Here's how the part is built. I have some questions about the finished solid (model axes, mm). Face numbers are marked on the shaded views. A direction names the side the tool comes from. Give positions to 0.01 mm unless a question says otherwise; leave off trailing zeros. Write each loop counter-clockwise with the first axis right and the second up, starting at its lowest first coordinate (ties: lowest second). Pieces come first, ordered by that corner, then holes. Notation, with made-up numbers: (79.25, 54.25) - (86.25, 54.25) arc R20 cw to (86.25, 73.25) - close; hole circle Ø6 at (42, 22.5). An arc over 180 degrees is marked (long way). Write each question's results on one line, items separated by ' | '. Start each with the question number.
Item 1: We'd pull the mould along Y, two halves only. Please class the marked faces 1, 2, 3 and 4: +Y half, -Y half, draft (parallel to the pull), parting line (faces both ways), or undercut.
Item 2: Suppose I cut it at A-A on z = 3.5. List the corners of the cut face in (x, y) for me, then the cut area to 3 significant figures.
Item 3: Which directions (+Z, -Z, +X, -X, +Y, -Y) give clear straight access to the entire face, cutting with the end or side of a thin tool? Please do the marked faces 5 and 6.
Item 4: Will these pins go through, and if not, where does the flat tip stop? P1, Ø15, axis at x = 18, y = 31, coming from the -Z side; P2, Ø8, axis at x = 23.5, y = 22.5, coming from the -Z side; P3, Ø2.5, axis at x = 15.5, y = 8, coming from the -Z side.
Item 5: Suppose I cut it at C-C on y = 13.5. List the corners of the cut face in (x, z) for me, then the cut area to 3 significant figures.
Item 6: Suppose I cut it at B-B on x = 26. List the corners of the cut face in (y, z) for me, then the cut area to 3 significant figures.
Item 7: Please list where these lines run through material, in increasing order: line 1 along Y through (x, z) = (11.5, 12); line 2 along X through (y, z) = (18, 6.5); line 3 along Y through (x, z) = (27, 8.5).
```python
from build123d import *

# Parameters (mm, degrees)
SKETCH_1_W          = 33
SKETCH_1_H          = 44
EXTRUDE_1_DEPTH     = 12.5
SKETCH_2_W          = 29.6
SKETCH_2_H          = 40.6
CUT_EXTRUDE_2_DEPTH = 11
SKETCH_3_W          = 27.6
SKETCH_3_H          = 31.1
CUT_EXTRUDE_3_DEPTH = 2.5
SKETCH_4_W          = 18
SKETCH_4_H          = 3
CUT_EXTRUDE_4_DEPTH = 0.7
FILLET_1_R          = 1
SKETCH_5_W          = 27.6
SKETCH_5_H          = 0.6
EXTRUDE_2_DEPTH     = 1
EXTRUDE_3_DEPTH     = 8
EXTRUDE_4_DEPTH     = 0.6
SKETCH_8_W          = 27.6
SKETCH_8_H          = 27.1
CUT_EXTRUDE_5_DEPTH = 1.6
CUT_EXTRUDE_6_DEPTH = 5


with BuildPart() as part:
    # 草图1 → 凸台-拉伸1 (new body)
    with BuildSketch(Plane.XY):
        with Locations((16.5, 22)):
            Rectangle(SKETCH_1_W, SKETCH_1_H)
    extrude(amount=EXTRUDE_1_DEPTH)

    # 草图2 → 切除-拉伸2 (cut)
    with BuildSketch(Plane(origin=(0, 0, 0), x_dir=(-1, 0, 0), z_dir=(0, 0, -1))):
        with Locations((-16.5, 22)):
            Rectangle(SKETCH_2_W, SKETCH_2_H)
    extrude(amount=-CUT_EXTRUDE_2_DEPTH, mode=Mode.SUBTRACT)

    # 草图3 → 切除-拉伸3 (cut, through all)
    with BuildSketch(Plane(origin=(0, 0, 11), x_dir=(-1, 0, 0), z_dir=(0, 0, -1))):
        with Locations((-16.5, 21.75)):
            Rectangle(SKETCH_3_W, SKETCH_3_H)
    extrude(amount=-CUT_EXTRUDE_3_DEPTH, mode=Mode.SUBTRACT)

    # 草图4 → 切除-拉伸4 (cut)
    with BuildSketch(Plane(origin=(0, 0, 11), x_dir=(-1, 0, 0), z_dir=(0, 0, -1))):
        with Locations((-16.5, 40.8)):
            Rectangle(SKETCH_4_W, SKETCH_4_H)
    extrude(amount=-CUT_EXTRUDE_4_DEPTH, mode=Mode.SUBTRACT)

    # 圆角1
    fillet_1_edges = [part.edges().sort_by_distance(p)[0] for p in [
        (0, 44, 6.25),
        (33, 44, 6.25),
        (33, 0, 6.25),
        (0, 0, 6.25),
    ]]
    fillet(fillet_1_edges, radius=FILLET_1_R)

    # 草图5 → 凸台-拉伸2 (add)
    with BuildSketch(Plane(origin=(0, 6.2, 0), x_dir=(1, 0, 0), z_dir=(0, 1, 0))):
        with Locations((16.5, -12.2)):
            Rectangle(SKETCH_5_W, SKETCH_5_H)
    extrude(amount=EXTRUDE_2_DEPTH)

    # 草图6 → 凸台-拉伸3 (add)
    with BuildSketch(Plane(origin=(0, 0, 11), x_dir=(-1, 0, 0), z_dir=(0, 0, -1))):
        with BuildLine():
            Line((-31.3, 11.6), (-31.3, 12.4))
            ThreePointArc((-31.3, 12.4), (-30.9, 12), (-31.3, 11.6))
        make_face()
        with BuildLine():
            Line((-31.3, 32.4), (-31.3, 31.6))
            ThreePointArc((-31.3, 31.6), (-30.9, 32), (-31.3, 32.4))
        make_face()
        with BuildLine():
            Line((-28.8, 42.3), (-28, 42.3))
            ThreePointArc((-28, 42.3), (-28.4, 41.9), (-28.8, 42.3))
        make_face()
        with BuildLine():
            Line((-28.8, 1.7), (-28, 1.7))
            ThreePointArc((-28, 1.7), (-28.4, 2.1), (-28.8, 1.7))
        make_face()
        with BuildLine():
            Line((-4.2, 1.7), (-5, 1.7))
            ThreePointArc((-5, 1.7), (-4.6, 2.1), (-4.2, 1.7))
        make_face()
        with BuildLine():
            Line((-4.2, 42.3), (-5, 42.3))
            ThreePointArc((-5, 42.3), (-4.6, 41.9), (-4.2, 42.3))
        make_face()
        with BuildLine():
            Line((-1.7, 32.4), (-1.7, 31.6))
            ThreePointArc((-1.7, 31.6), (-2.1, 32), (-1.7, 32.4))
        make_face()
        with BuildLine():
            Line((-1.7, 11.6), (-1.7, 12.4))
            ThreePointArc((-1.7, 12.4), (-2.1, 12), (-1.7, 11.6))
        make_face()
    extrude(amount=EXTRUDE_3_DEPTH)

    # 草图7 → 凸台-拉伸4 (add)
    with BuildSketch(Plane.XY.offset(12.5)):
        with BuildLine():
            Line((0, 43), (0, 1))
            ThreePointArc((0, 1), (0.292893219, 0.292893219), (1, 0))
            Line((1, 0), (32, 0))
            ThreePointArc((32, 0), (32.707106781, 0.292893219), (33, 1))
            Line((33, 1), (33, 43))
            ThreePointArc((33, 43), (32.707106781, 43.707106781), (32, 44))
            Line((32, 44), (1, 44))
            ThreePointArc((1, 44), (0.292893219, 43.707106781), (0, 43))
        make_face()
    extrude(amount=EXTRUDE_4_DEPTH)

    # 草图8 → 切除-拉伸5 (cut, through all)
    with BuildSketch(Plane(origin=(0, 0, 12.5), x_dir=(-1, 0, 0), z_dir=(0, 0, -1))):
        with Locations((-16.5, 23.75)):
            Rectangle(SKETCH_8_W, SKETCH_8_H)
    extrude(amount=-CUT_EXTRUDE_5_DEPTH, mode=Mode.SUBTRACT)

    # 草图9 → 切除-拉伸6 (cut)
    with BuildSketch(Plane(origin=(0, 34.3, 0), x_dir=(-1, 0, 0), z_dir=(0, -1, 0))):
        Polygon((-31.3, -1.2), (-32.1, -2), (-31.3, -2.8), align=None)
        Polygon((-1.7, -2.8), (-1.7, -1.2), (-0.9, -2), align=None)
    cut_extrude_6 = extrude(amount=-CUT_EXTRUDE_6_DEPTH, mode=Mode.SUBTRACT)

    # 镜向1: 切除-拉伸6 across plane
    add(cut_extrude_6.mirror(Plane(origin=(0, 22, 0), x_dir=(0, 0, 1), z_dir=(0, -1, 0))), mode=Mode.SUBTRACT)


solid = part.part
```
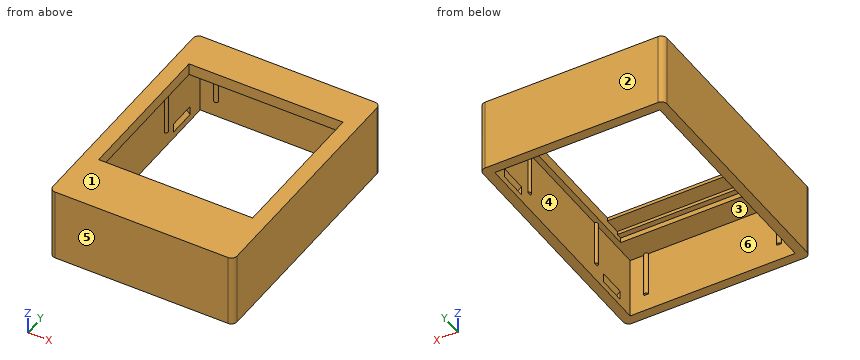
Checked values:
1) face 1: draft | face 2: +Y half | face 3: undercut | face 4: undercut
2) outline: (0, 1) arc R1 ccw to (1, 0) - (32, 0) arc R1 ccw to (33, 1) - (33, 43) arc R1 ccw to (32, 44) - (1, 44) arc R1 ccw to (0, 43) - close; hole (1.7, 1.7) - (4.2, 1.7) arc R0.4 cw to (5, 1.7) - (28, 1.7) arc R0.4 cw to (28.8, 1.7) - (31.3, 1.7) - (31.3, 11.6) arc R0.4 cw to (31.3, 12.4) - (31.3, 31.6) arc R0.4 cw to (31.3, 32.4) - (31.3, 42.3) - (28.8, 42.3) arc R0.4 cw to (28, 42.3) - (5, 42.3) arc R0.4 cw to (4.2, 42.3) - (1.7, 42.3) - (1.7, 32.4) arc R0.4 cw to (1.7, 31.6) - (1.7, 12.4) arc R0.4 cw to (1.7, 11.6) - close | area: 251 mm^2
3) face 5: +Z, -Z, +X, -X, -Y | face 6: -Z
4) P1: stops at z = 11 | P2: passes through | P3: stops at z = 11.9
5) outline: (0, 0) - (1.7, 0) - (1.7, 11) - (2.7, 11) - (2.7, 13.1) - (0, 13.1) - close; (30.3, 11) - (31.3, 11) - (31.3, 0) - (33, 0) - (33, 13.1) - (30.3, 13.1) - close | area: 48.7 mm^2
6) outline: (0, 0) - (1.7, 0) - (1.7, 11) - (6.2, 11) - (6.2, 11.9) - (7.2, 11.9) - (7.2, 12.5) - (10.2, 12.5) - (10.2, 13.1) - (0, 13.1) - close; (37.3, 11) - (42.3, 11) - (42.3, 0) - (44, 0) - (44, 13.1) - (37.3, 13.1) - close | area: 67.5 mm^2
7) line 1: y = 0 to 7.2, 37.3 to 44 | line 2: x = 0 to 1.7, 31.3 to 33 | line 3: y = 0 to 1.7, 42.3 to 44
